```python
from build123d import *

# Parameters (mm, degrees)
SKETCH1_R           = 1.65
BOSS_EXTRUDE3_DEPTH = 3
FILLET1_R           = 2.54
SKETCH6_R           = 6.35
BUTTONS_DEPTH       = 4
SKETCH7_R           = 1.75
CUT_EXTRUDE5_DEPTH  = 4
SKETCH8_W           = 4.318
SKETCH8_H           = 8.636
CUT_EXTRUDE6_DEPTH  = 4


with BuildPart() as part:
    # Sketch1 → Boss-Extrude3 (new body)
    with BuildSketch(Plane(origin=(0, 0, 0), x_dir=(1, 0, 0), z_dir=(0, 1, 0))):
        with BuildLine():
            Line((48.284490735, 53.109977813), (-64.735509285, 53.109977813))
            Line((-64.735509285, 53.109977813), (-64.735509285, -72.290076187))
            Line((-64.735509285, -72.290076187), (22.884490735, -72.290076187))
            ThreePointArc((22.884490735, -72.290076187), (40.845002977, -64.850588429), (48.284490735, -46.890076187))
            Line((48.284490735, -46.890076187), (48.284490735, 53.109977813))
        make_face()
        with Locations((-59.655509285, 48.029977813)):
            Circle(SKETCH1_R, mode=Mode.SUBTRACT)
        with Locations((43.204490735, 48.029977813)):
            Circle(SKETCH1_R, mode=Mode.SUBTRACT)
        with Locations((-59.655509285, -67.210076187)):
            Circle(SKETCH1_R, mode=Mode.SUBTRACT)
        with Locations((37.880892571, -60.748479124)):
            Circle(SKETCH1_R, mode=Mode.SUBTRACT)
    extrude(amount=BOSS_EXTRUDE3_DEPTH)

    # Fillet1
    fillet1_edges = [part.edges().sort_by_distance(p)[0] for p in [
        (-64.735509285, 1.5, 72.290076187),
        (-64.735509285, 1.5, -53.109977813),
        (48.284490735, 1.5, -53.109977813),
    ]]
    fillet(fillet1_edges, radius=FILLET1_R)

    # Sketch6 → Buttons (cut, through all)
    with BuildSketch(Plane(origin=(0, 3, 0), x_dir=(1, 0, 0), z_dir=(0, 1, 0))):
        with Locations((22.884490735, 13.109977813)):
            Circle(SKETCH6_R)
        with Locations((22.884490735, -2.890022187)):
            Circle(SKETCH6_R)
        with Locations((22.884490735, -18.890022187)):
            Circle(SKETCH6_R)
        with Locations((22.884490735, -34.890022187)):
            Circle(SKETCH6_R)
        with Locations((22.884490735, -50.890022187)):
            Circle(SKETCH6_R)
    extrude(amount=-BUTTONS_DEPTH, mode=Mode.SUBTRACT)

    # Sketch7 → Cut-Extrude5 (cut, through all)
    with BuildSketch(Plane(origin=(0, 3, 0), x_dir=(1, 0, 0), z_dir=(0, 1, 0))):
        with Locations((28.284490735, 41.109977813)):
            Circle(SKETCH7_R)
        with Locations((28.284490735, 33.489977813)):
            Circle(SKETCH7_R)
        with Locations((28.284490735, 25.869977813)):
            Circle(SKETCH7_R)
    extrude(amount=-CUT_EXTRUDE5_DEPTH, mode=Mode.SUBTRACT)

    # Sketch8 → Cut-Extrude6 (cut, through all)
    with BuildSketch(Plane(origin=(0, 3, 0), x_dir=(1, 0, 0), z_dir=(0, 1, 0))):
        with Locations((-49.556509265, 33.791977813)):
            Rectangle(SKETCH8_W, SKETCH8_H)
    extrude(amount=-CUT_EXTRUDE6_DEPTH, mode=Mode.SUBTRACT)


solid = part.part
```
Input: part model. Units: mm. Frame: model coordinates. A direction names the side the tool comes from. Give positions to 0.01 mm unless a question says otherwise; leave off trailing zeros. Write each loop counter-clockwise with the first axis right and the second up, starting at its lowest first coordinate (ties: lowest second). Pieces come first, ordered by that corner, then holes. Notation, with made-up numbers: (58, 40) - (115, 40) arc R16 cw to (115, 45) - close; hole circle Ø3 at (-27, 64.5). An arc over 180 degrees is marked (long way). Write item = value, one per line. Start each with the question number.
1) Pin query (flat end, axial travel): pin 1 (20.5 mm diameter, centred on x = 22.88, z = 18.89, fed in from -Y); pin 2 (2 mm diameter, centred on x = 37.88, z = 60.75, fed in from +Y). Return the tip coordinate at first contact, or that it passes through.
2) Cut plane A-A (z = 49). Return loops of the section in (x, y), and give its area (3 significant figures).
3) Reachability of faces 1 (the face through (-51.716, 2, -34)), 2 (the face through (-64.01, 1.52, 71.53)) from +Z, -Z, +X, -X, +Y, -Y: full face, straight path, thin tool, end or side. Return the list, or none.
4) Cut plane B-B (y = 0.5). Give the number of separate pieces and of enclosed holes in the cut face, and give its area (3 significant figures).
5) Cut plane C-C (z = -2). Return loops of the section in (x, y).
6) Draft query along Z for faces 3 (the face through (18.204, 1.521, -17.402)), 4 (the face through (-9, 0, 9)), 5 (the face through (27.91, 1.52, -24.16)), 6 (the face through (-63.97, 1.52, -52.39)). Return one class per face: pulls with the +Z half, pulls with the -Z half, needs draft (parallel to the pull), parting line crosses it, or undercut.
7) Material intervals for L1, parallel to Z at x = 24.5, y = 0.7; L2, parallel to Z at x = 43.5, y = 2.95; L3, parallel to X at y = 2.4, z = 0, sorted ascending. Write a range as [from, to].
Answers follow:
q1.pin_1 = 0
q1.pin_2 = through
q2.outline = (-64.74, 0) - (16.82, 0) - (16.82, 3) - (-64.74, 3) - close; (28.95, 0) - (48.2, 0) - (48.2, 3) - (28.95, 3) - close
q2.area = 302 mm^2
q3.face_1 = +Y, -Y
q3.face_2 = +Z, -X, +Y, -Y
q4.separate_pieces = 1
q4.enclosed_holes = 13
q4.area = 13,300 mm^2
q5.outline = (-64.74, 0) - (18.83, 0) - (18.83, 3) - (-64.74, 3) - close; (26.94, 0) - (48.28, 0) - (48.28, 3) - (26.94, 3) - close
q6.face_3 = undercut
q6.face_4 = needs draft
q6.face_5 = undercut
q6.face_6 = pulls with the -Z half
q7.L1 = [-53.11, -19.25], [-6.97, -3.25], [9.03, 12.75], [25.03, 28.75], [41.03, 44.75], [57.03, 72.24]
q7.L2 = [-53.11, -49.65], [-46.41, 61.73]
q7.L3 = [-64.74, 17.23], [28.54, 48.28]
